Geometry check sheet. Reference: drawing and pictorial views, mm from the part's lowest x, y, z. Give positions to 0.01 mm unless a question says otherwise; leave off trailing zeros. Order: outer loops, then holes, each group sorted by start corner. A loop starts at its lowest first (then second) coordinate and runs counter-clockwise, first axis right, second up.
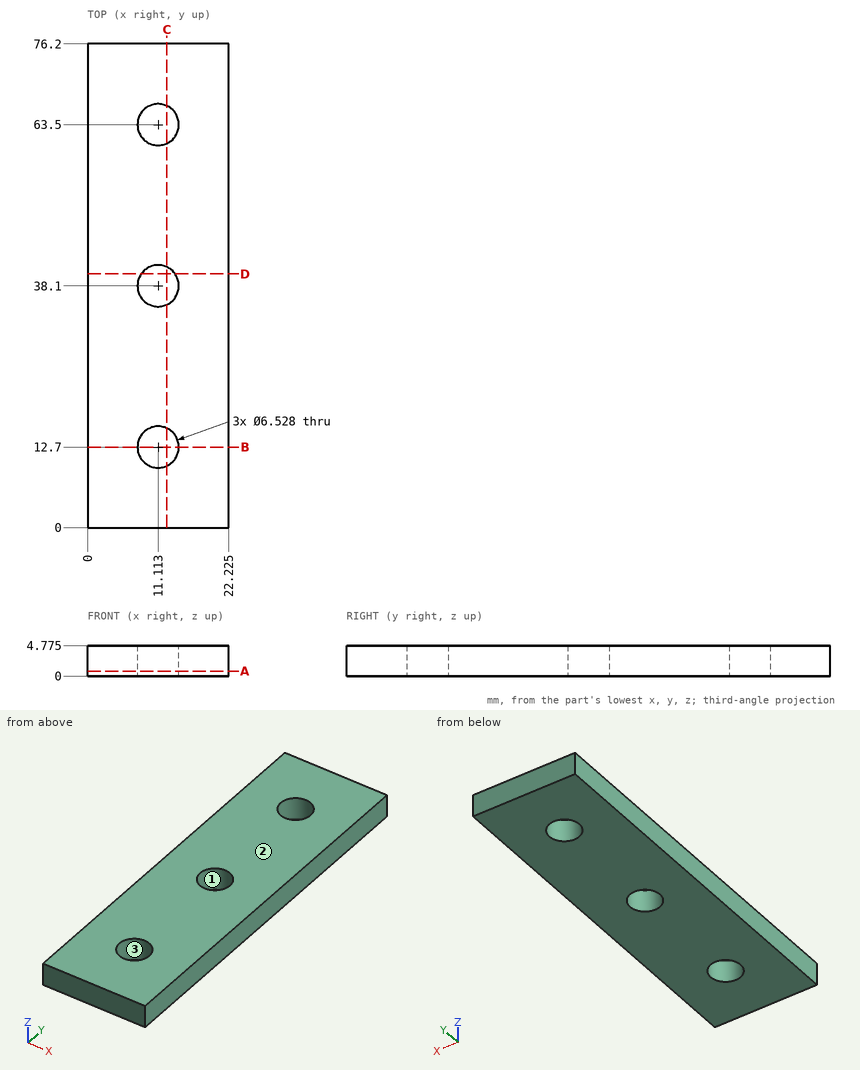
(1) Sectioned sample at B-B (y = 12.7). Enter the section's corners in (x, z) (1 decimal).
(2) Sectioned sample at D-D (y = 40). Enter the section's corners in (x, z) (1 decimal).
(3) Release check for a two-part mould opening along X. For the marked faces 1, 2 and 3 record: released by +X, released by -X, zero draft, split by the parting line, or undercut.
(4) Sectioned sample at C-C (x = 12.5). Enter the section's corners in (y, z) (1 decimal), plus the area to 3 significant figures.
(5) Go/stop test with a flat-tipped pin: P1, Ø4, axis at x = 9.5, y = 29.5, coming from the -Z side. Record where the tip stops, or that it passes through.
(6) Thickness scan on L1, parallel to Y at x = 11.25, z = 1.4; L2, parallel to Y at x = 8.25, z = 4.3 (1 decimal); L3, parallel to X at y = 37.5, z = 3.9 (1 decimal). Record the ranges inside material, lowest first.
(7) Sectioned sample at A-A (z = 0.75). Enter the section's corners in (x, y) (1 decimal), plus the area to 3 significant figures.
Values follow:
1. outline: (0, 0) - (7.8, 0) - (7.8, 4.8) - (0, 4.8) - close; (14.4, 0) - (22.2, 0) - (22.2, 4.8) - (14.4, 4.8) - close
2. outline: (0, 0) - (8.5, 0) - (8.5, 4.8) - (0, 4.8) - close; (13.8, 0) - (22.2, 0) - (22.2, 4.8) - (13.8, 4.8) - close
3. face 1: undercut
3. face 2: zero draft
3. face 3: undercut
4. outline: (0, 0) - (9.7, 0) - (9.7, 4.8) - (0, 4.8) - close; (15.7, 0) - (35.1, 0) - (35.1, 4.8) - (15.7, 4.8) - close; (41.1, 0) - (60.5, 0) - (60.5, 4.8) - (41.1, 4.8) - close; (66.5, 0) - (76.2, 0) - (76.2, 4.8) - (66.5, 4.8) - close
4. area: 279 mm2
5. P1: stops at z = 0
6. L1: y = 0 to 9.44, 15.96 to 34.84, 41.36 to 60.24, 66.76 to 76.2
6. L2: y = 0 to 11.1, 14.3 to 36.5, 39.7 to 61.9, 65.1 to 76.2
6. L3: x = 0 to 7.9, 14.3 to 22.2
7. outline: (0, 0) - (22.2, 0) - (22.2, 76.2) - (0, 76.2) - close; hole circle Ø6.5 at (11.1, 12.7); hole circle Ø6.5 at (11.1, 38.1); hole circle Ø6.5 at (11.1, 63.5)
7. area: 1,590 mm2
